```python
from build123d import *

# Parameters (mm, degrees)
SKETCH1_W           = 28
SKETCH1_H           = 30
SKETCH1_R           = 11.1
SKETCH1_R_2         = 1.6
BOSS_EXTRUDE1_DEPTH = 7
SKETCH1_4_R         = 1.6
CUT_EXTRUDE3_DEPTH  = 3
FILLET5_R           = 4


with BuildPart() as part:
    # Sketch1 → Boss-Extrude1 (new body)
    with BuildSketch(Plane.XY):
        Rectangle(SKETCH1_W, SKETCH1_H)
        Circle(SKETCH1_R, mode=Mode.SUBTRACT)
        with Locations((-10.234773755, 10.965829024)):
            Circle(SKETCH1_R_2, mode=Mode.SUBTRACT)
        with Locations((10.234773755, 10.965829024)):
            Circle(SKETCH1_R_2, mode=Mode.SUBTRACT)
        with Locations((-10.234773755, -10.965829024)):
            Circle(SKETCH1_R_2, mode=Mode.SUBTRACT)
        with Locations((10.234773755, -10.965829024)):
            Circle(SKETCH1_R_2, mode=Mode.SUBTRACT)
    extrude(amount=BOSS_EXTRUDE1_DEPTH)

    # Sketch1_4 → Cut-Extrude3 (cut)
    # profile 1 of 4: a face of its own
    with BuildSketch(Plane.XY):
        Polygon((10.234773755, 7.617197462), (7.334773755, 9.291513243), (7.334773755, 12.640144804), (10.234773755, 14.314460585), (13.134773755, 12.640144804), (13.134773755, 9.291513243), align=None)
        with Locations((10.234773755, 10.965829024)):
            Circle(SKETCH1_4_R, mode=Mode.SUBTRACT)
    # profile 2 of 4: a face of its own
    with BuildSketch(Plane.XY):
        Polygon((-13.134773755, 12.640144804), (-13.134773755, 9.291513243), (-10.234773755, 7.617197462), (-7.334773755, 9.291513243), (-7.334773755, 12.640144804), (-10.234773755, 14.314460585), align=None)
        with Locations((-10.234773755, 10.965829024)):
            Circle(SKETCH1_4_R, mode=Mode.SUBTRACT)
    # profile 3 of 4: a face of its own
    with BuildSketch(Plane.XY):
        Polygon((-13.134773755, -9.291513243), (-10.234773755, -7.617197462), (-7.334773755, -9.291513243), (-7.334773755, -12.640144804), (-10.234773755, -14.314460585), (-13.134773755, -12.640144804), align=None)
        with Locations((-10.234773755, -10.965829024)):
            Circle(SKETCH1_4_R, mode=Mode.SUBTRACT)
    # profile 4 of 4: a face of its own
    with BuildSketch(Plane.XY):
        Polygon((13.134773755, -9.291513243), (10.234773755, -7.617197462), (7.334773755, -9.291513243), (7.334773755, -12.640144804), (10.234773755, -14.314460585), (13.134773755, -12.640144804), align=None)
        with Locations((10.234773755, -10.965829024)):
            Circle(SKETCH1_4_R, mode=Mode.SUBTRACT)
    extrude(amount=CUT_EXTRUDE3_DEPTH, mode=Mode.SUBTRACT)

    # Fillet5
    fillet5_edges = [part.edges().sort_by_distance(p)[0] for p in [
        (14, -15, 3.5),
        (-14, -15, 3.5),
        (-14, 15, 3.5),
        (14, 15, 3.5),
    ]]
    fillet(fillet5_edges, radius=FILLET5_R)


solid = part.part
```
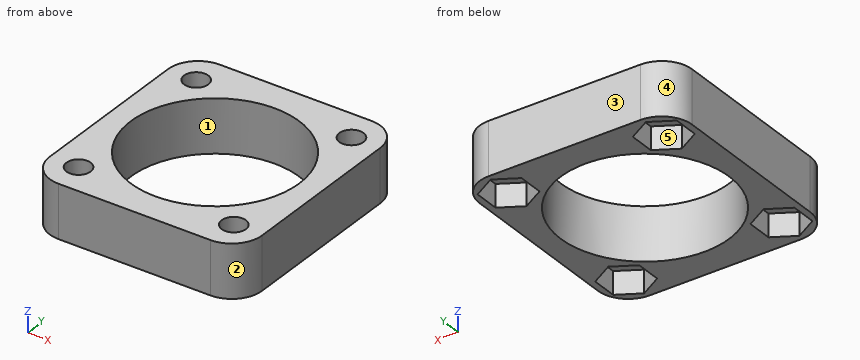
Part model, mm, in its own coordinate system. Face numbers are marked on the shaded views. A direction names the side the tool comes from. Coordinates: 2 decimals unless noted, no trailing zeros. Write each loop counter-clockwise with the first axis right and the second up, starting at its lowest first coordinate (ties: lowest second). Pieces come first, ordered by that corner, then holes.
Item 1: Mould opens along Y. For the marked faces 1, 2 and 3 say: released by +Y, released by -Y, zero draft, split by the parting line, or undercut.
Item 2: Slice it at A-A (y = 0). Write the cut outline in (x, z).
Item 3: Slice it at C-C (z = 1.25). Count the separate pieces of the cut face and the enclosed holes in it, and give its area (3 significant figures).
Item 4: Probe line 1 (Y direction, x = 0, z = 4.25); line 2 (Y direction, x = 10, z = 1); line 3 (X direction, y = 11.5, z = 6.5). List the from-to ranges inside material, lowest first.
Item 5: Pin check, flat tips, straight feed: pin 1 (10 mm diameter, centred on x = 2.5, y = 5.5, fed in from +Z); pin 2 (1.7 mm diameter, centred on x = -10, y = 12, fed in from -Z). Stop position of each tip, or through.
Item 6: Which spindle directions (+Z, -Z, +X, -X, +Y, -Y) get a long thin tool onto all of the face, cutting with end or side? Do the marked faces 4 and 5. Say none if no direction does.
Item 7: Slice it at B-B (x = 0). Write the cut outline in (y, z).
Item 8: Slice it at D-D (y = 10). Write the cut outline in (x, z), and give its area (3 significant figures).
Results found:
1. face 1: undercut
1. face 2: released by -Y
1. face 3: released by +Y
2. outline: (-14, 0) - (-11.1, 0) - (-11.1, 7) - (-14, 7) - close; (11.1, 0) - (14, 0) - (14, 7) - (11.1, 7) - close
3. separate pieces: 1
3. enclosed holes: 5
3. area: 323 mm2
4. line 1: y = -15 to -11.1, 11.1 to 15
4. line 2: y = -15 to -14.18, -7.75 to -4.82, 4.82 to 7.75, 14.18 to 15
4. line 3: x = -13.97 to -11.74, -8.73 to 8.73, 11.74 to 13.97
5. pin 1: passes through
5. pin 2: stops at z = 3
6. face 4: +Z, -Z, -X, +Y
6. face 5: -Z
7. outline: (-15, 0) - (-11.1, 0) - (-11.1, 7) - (-15, 7) - close; (11.1, 0) - (15, 0) - (15, 7) - (11.1, 7) - close
8. outline: (-14, 0) - (-13.13, 0) - (-13.13, 3) - (-11.51, 3) - (-11.51, 7) - (-14, 7) - close; (-8.96, 3) - (-7.33, 3) - (-7.33, 0) - (-4.82, 0) - (-4.82, 7) - (-8.96, 7) - close; (4.82, 0) - (7.33, 0) - (7.33, 3) - (8.96, 3) - (8.96, 7) - (4.82, 7) - close; (11.51, 3) - (13.13, 3) - (13.13, 0) - (14, 0) - (14, 7) - (11.51, 7) - close
8. area: 73.3 mm2
